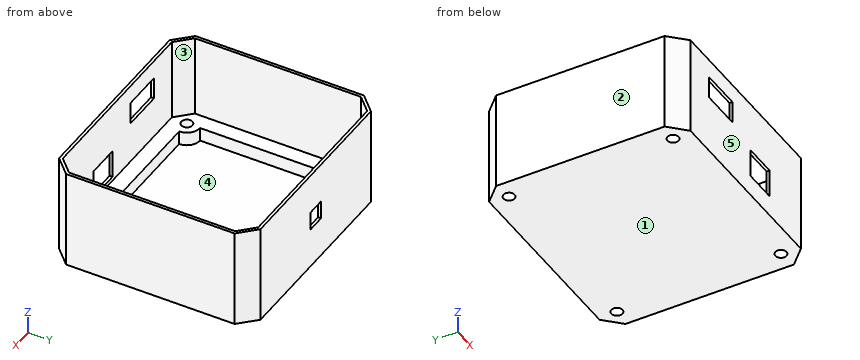
from build123d import *

# Parameters (mm, degrees)
EXTRUDE_1_DEPTH     = 22.2
EXTRUDE_2_DEPTH     = 4.5
SKETCH_3_R          = 1.5
CUT_EXTRUDE_1_DEPTH = 47.223181414
CUT_EXTRUDE_3_DEPTH = 3.7
CUT_EXTRUDE_4_REACH = 67.816
SKETCH_6_W          = 9
SKETCH_6_H          = 7.6
SKETCH_6_W_2        = 11
SKETCH_6_H_2        = 6
CUT_EXTRUDE_5_REACH = 67.816
SKETCH_7_W          = 5
SKETCH_7_H          = 5


with BuildPart() as part:
    # 草圖1 → 填料-伸長1 (new body)
    with BuildSketch(Plane.XY):
        Polygon((-25.794213562, 27.05), (25.794213562, 27.05), (30.2, 22.644213562), (30.2, -22.644213562), (25.794213562, -27.05), (-25.794213562, -27.05), (-30.2, -22.644213562), (-30.2, 22.644213562), align=None)
        Polygon((-29.4, 22.312842712), (-25.462842712, 26.25), (25.462842712, 26.25), (29.4, 22.312842712), (29.4, -22.312842712), (25.462842712, -26.25), (-25.462842712, -26.25), (-29.4, -22.312842712), align=None, mode=Mode.SUBTRACT)
    extrude(amount=EXTRUDE_1_DEPTH)

    # 草圖2 → 填料-伸長2 (add)
    with BuildSketch(Plane(origin=(0, 0, 0), x_dir=(-1, 0, 0), z_dir=(0, 0, -1))):
        Polygon((-30.2, 22.644213562), (-25.794213562, 27.05), (25.794213562, 27.05), (30.2, 22.644213562), (30.2, -22.644213562), (25.794213562, -27.05), (-25.794213562, -27.05), (-30.2, -22.644213562), align=None)
    extrude(amount=EXTRUDE_2_DEPTH)

    # 草圖3 → 除料-伸長1 (cut, through all)
    with BuildSketch(Plane.XY):
        with Locations((25.2, 22.03)):
            Circle(SKETCH_3_R)
        with Locations(Location((25.2, -22.03, 0), (0, 0, 180))):
            Circle(SKETCH_3_R)
        with Locations((-25.2, -22.03)):
            Circle(SKETCH_3_R)
        with Locations(Location((-25.2, 22.03, 0), (0, 0, 180))):
            Circle(SKETCH_3_R)
    extrude(amount=-CUT_EXTRUDE_1_DEPTH, mode=Mode.SUBTRACT)

    # 草圖5 → 除料-伸長3 (cut)
    with BuildSketch(Plane.XY):
        with BuildLine():
            Line((-25.234050993, 18.530165643), (-25.234050993, -18.530165643))
            ThreePointArc((-25.234050993, -18.530165643), (-22.715358839, -19.564932394), (-21.700544406, -22.091729589))
            Line((-21.700544406, -22.091729589), (21.700544406, -22.091729589))
            ThreePointArc((21.700544406, -22.091729589), (22.737758998, -19.542557689), (25.297360416, -18.531354412))
            Line((25.297360416, -18.531354412), (25.297360416, 18.531354412))
            ThreePointArc((25.297360416, 18.531354412), (22.56426249, 19.727200014), (21.74608079, 22.596076045))
            Line((21.74608079, 22.596076045), (-21.74608079, 22.596076045))
            ThreePointArc((-21.74608079, 22.596076045), (-22.543539666, 19.751136578), (-25.234050993, 18.530165643))
        make_face()
    extrude(amount=-CUT_EXTRUDE_3_DEPTH, mode=Mode.SUBTRACT)

    # 草圖6 → 除料-伸長4 (cut, up to next)
    with BuildSketch(Plane.XZ.offset(27.05), mode=Mode.PRIVATE) as cut_extrude_4_sk1:
        with Locations((6.7, 4.9)):
            Rectangle(SKETCH_6_W, SKETCH_6_H)
    cut_extrude_4_tool1 = extrude(cut_extrude_4_sk1.sketch, amount=-CUT_EXTRUDE_4_REACH, mode=Mode.PRIVATE) & part.part
    # 草圖6 → 除料-伸長4 (cut, up to next)
    with BuildSketch(Plane.XZ.offset(27.05), mode=Mode.PRIVATE) as cut_extrude_4_sk2:
        with Locations((-11.7, 14.2)):
            Rectangle(SKETCH_6_W_2, SKETCH_6_H_2)
    cut_extrude_4_tool2 = extrude(cut_extrude_4_sk2.sketch, amount=-CUT_EXTRUDE_4_REACH, mode=Mode.PRIVATE) & part.part
    add(cut_extrude_4_tool1.solids().sort_by_distance((6.7, -27.05, 4.9))[0], mode=Mode.SUBTRACT)
    add(cut_extrude_4_tool2.solids().sort_by_distance((-11.7, -27.05, 14.2))[0], mode=Mode.SUBTRACT)

    # 草圖7 → 除料-伸長5 (cut, up to next)
    with BuildSketch(Plane(origin=(0, 27.05, 0), x_dir=(1, 0, 0), z_dir=(0, 1, 0)), mode=Mode.PRIVATE) as cut_extrude_5_sk1:
        with Locations((0, -8.85)):
            Rectangle(SKETCH_7_W, SKETCH_7_H)
    cut_extrude_5_tool1 = extrude(cut_extrude_5_sk1.sketch, amount=-CUT_EXTRUDE_5_REACH, mode=Mode.PRIVATE) & part.part
    add(cut_extrude_5_tool1.solids().sort_by_distance((0, 27.05, 8.85))[0], mode=Mode.SUBTRACT)


solid = part.part
Check sheet for the modelled part. Datum: model origin and axes. Units: mm. Face numbers are marked on the shaded views. A direction names the side the tool comes from. Round coordinates to 2 decimals unless told otherwise and drop trailing zeros. Loops run counter-clockwise (first coordinate to the right, second up) from the corner with the lowest first, then second, coordinate; pieces in that order, holes last. Notation, with made-up numbers: (-11, -28.5) - (14, -28.5) arc R22 cw to (14, -20.5) - close; hole circle Ø11 at (88.25, 9.5). An arc over 180 degrees is marked (long way). Answer as CSV lines item,"result". Start each with the question number.
Item 1: Release check for a two-part mould opening along X. For the marked faces 1, 2 and 3 record: +X half, -X half, draft (parallel to the pull), parting line (faces both ways), or undercut.
Item 2: Section check D-D (y = 12). Record the boundary of the cut face in (x, z).
Item 3: Scan lines: line 1 (Y direction, x = 25.2, z = -3.55); line 2 (X direction, y = 21.5, z = 20); line 3 (Y direction, x = -9.5, z = 0.5). Record each from-to range of solid material in increasing order. Write a range as [from, to].
Item 4: Set-up check for the marked faces 4 and 5: record each of +Z, -Z, +X, -X, +Y, -Y from which the full face is reachable in a straight line by a thin tool's end or side.
Item 5: Depth check by flat-ended pin: P1, Ø1, axis at x = 5.5, z = 2.5, coming from the -Y side; P2, Ø3, axis at x = 17, y = 19.5, coming from the +Z side; P3, Ø2.5, axis at x = -25.2, y = -22.03, coming from the -Z side; P4, Ø0.6, axis at y = -27, z = 15, coming from the +X side. Enter the tip coordinate at first touch or a pass-through.
Item 6: Section check C-C (z = -1). Record the boundary of the cut face in (x, y).
Item 7: Section check B-B (x = 0). Record the boundary of the cut face in (y, z), and give its area (3 significant figures).
Item 8: Section check A-A (z = 7.5). Record the boundary of the cut face in (x, y), and give its area (3 significant figures).
Report:
1,face 1,"draft"
1,face 2,"-X half"
1,face 3,"undercut"
2,outline,"(-30.2, -4.5) - (30.2, -4.5) - (30.2, 22.2) - (29.4, 22.2) - (29.4, 0) - (25.3, 0) - (25.3, -3.7) - (-25.23, -3.7) - (-25.23, 0) - (-29.4, 0) - (-29.4, 22.2) - (-30.2, 22.2) - close"
3,line 1,"y = [-27.05, -23.53], [-20.53, -18.53], [18.53, 20.53], [23.53, 27.05]"
3,line 2,"x = [-30.2, -29.4], [29.4, 30.2]"
3,line 3,"y = [-27.05, -26.25], [26.25, 27.05]"
4,face 4,"+Z"
4,face 5,"+Z, -Z, +X, -X, -Y"
5,P1,"stops at y = 26.25"
5,P2,"stops at z = -3.7"
5,P3,"passes through"
5,P4,"stops at x = 26.14"
6,outline,"(-30.2, -22.64) - (-25.79, -27.05) - (25.79, -27.05) - (30.2, -22.64) - (30.2, 22.64) - (25.79, 27.05) - (-25.79, 27.05) - (-30.2, 22.64) - close; hole circle Ø3 at (-25.2, -22.03); hole circle Ø3 at (-25.2, 22.03); hole (-25.23, -18.53) arc R3.5 cw to (-21.7, -22.09) - (21.7, -22.09) arc R3.5 cw to (25.3, -18.53) - (25.3, 18.53) arc R3.5 cw to (21.75, 22.6) - (-21.75, 22.6) arc R3.5 cw to (-25.23, 18.53) - close; hole circle Ø3 at (25.2, -22.03); hole circle Ø3 at (25.2, 22.03)"
7,outline,"(-27.05, -4.5) - (27.05, -4.5) - (27.05, 6.35) - (26.25, 6.35) - (26.25, 0) - (22.6, 0) - (22.6, -3.7) - (-22.09, -3.7) - (-22.09, 0) - (-26.25, 0) - (-26.25, 22.2) - (-27.05, 22.2) - close; (26.25, 11.35) - (27.05, 11.35) - (27.05, 22.2) - (26.25, 22.2) - close"
7,area,"110 mm2"
8,outline,"(-30.2, -22.64) - (-25.79, -27.05) - (2.2, -27.05) - (2.2, -26.25) - (-25.46, -26.25) - (-29.4, -22.31) - (-29.4, 22.31) - (-25.46, 26.25) - (-2.5, 26.25) - (-2.5, 27.05) - (-25.79, 27.05) - (-30.2, 22.64) - close; (2.5, 26.25) - (25.46, 26.25) - (29.4, 22.31) - (29.4, -22.31) - (25.46, -26.25) - (11.2, -26.25) - (11.2, -27.05) - (25.79, -27.05) - (30.2, -22.64) - (30.2, 22.64) - (25.79, 27.05) - (2.5, 27.05) - close"
8,area,"162 mm2"
